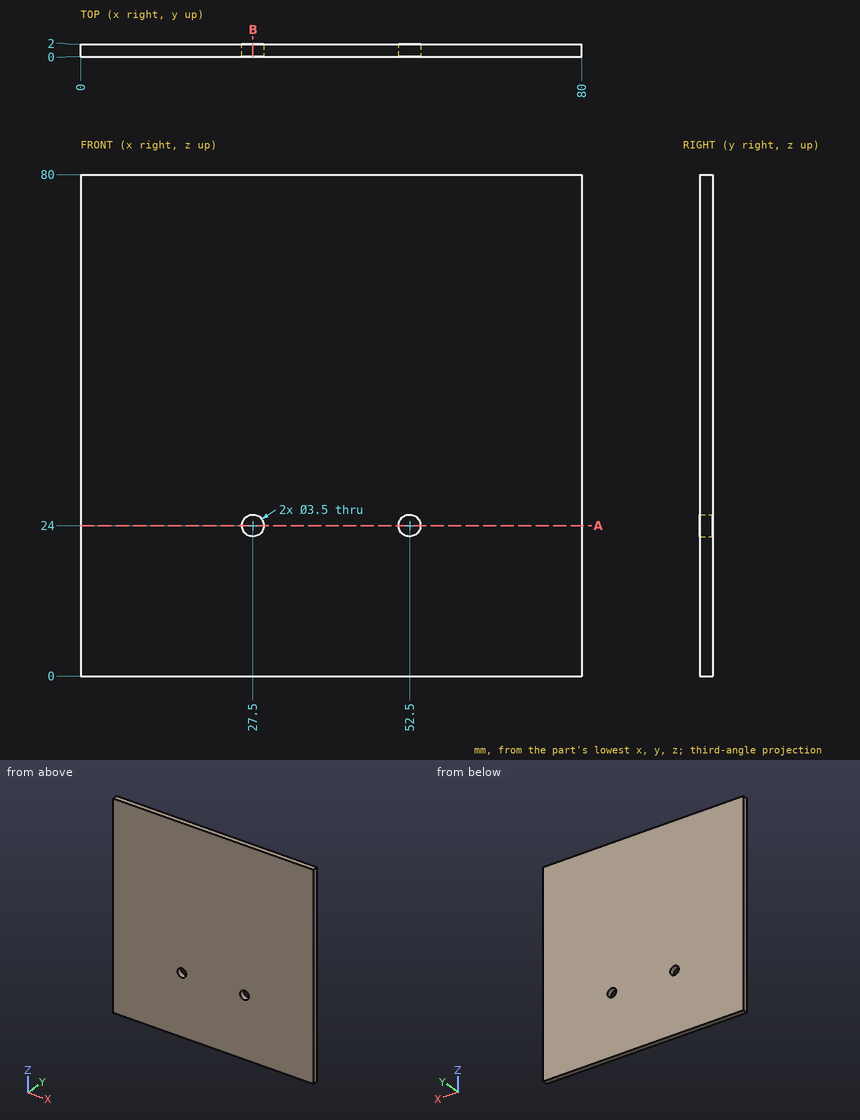
Verification items for this drawing (mm, ordinates from the low corner). Coordinates: 2 decimals unless noted, no trailing zeros. Write each loop counter-clockwise with the first axis right and the second up, starting at its lowest first coordinate (ties: lowest second). Pieces come first, ordered by that corner, then holes. Notation, with made-up numbers: M -8.5,24 L -4.5,24 A18 ccw -4.5,39 Z; hole C 85,69 d4. An arc over 180 degrees is marked long. Use one line per item in the form item = value. Start each with the question number.
1) Section check B-B on x = 27.5. Enter the section's corners in (y, z).
2) Thickness scan on probe 1 along X at (y, z) = (0.5, 24); probe 2 along Z at (x, y) = (27.5, 1.55); probe 3 along Z at (x, y) = (51, 0.85). Record the ranges inside material, lowest first. Write a range as from..to.
3) Section check A-A on z = 24. Enter the section's corners in (x, y).
4) Go/stop test with a flat-tipped pin: pin 1 Ø1 at (x, z) = (48.5, 53.5) entering from -Y. Record where the tip stops, or that it passes through.
Responses:
q1.outline = M 0,0 L 2,0 L 2,22.25 L 0,22.25 Z; M 0,25.75 L 2,25.75 L 2,80 L 0,80 Z
q2.probe_1 = 0..25.75, 29.25..50.75, 54.25..80
q2.probe_2 = 0..22.25, 25.75..80
q2.probe_3 = 0..23.1, 24.9..80
q3.outline = M 0,0 L 25.75,0 L 25.75,2 L 0,2 Z; M 29.25,0 L 50.75,0 L 50.75,2 L 29.25,2 Z; M 54.25,0 L 80,0 L 80,2 L 54.25,2 Z
q4.pin_1 = 0
